from build123d import *

# Parameters (mm, degrees)
SKETCH2_W                                      = 51.0032
SKETCH2_H                                      = 35.1028
BOSS_EXTRUDE1_DEPTH                            = 3.175
BOSS_EXTRUDE3_DEPTH                            = 12.7
M2X0_4_TAPPED_HOLE2_D                          = 1.6
CBORE_FOR_4_SOCKET_HEAD_CAP_SCREW4_D           = 3.2639
CBORE_FOR_4_SOCKET_HEAD_CAP_SCREW4_CBORE_D     = 5.55752
CBORE_FOR_4_SOCKET_HEAD_CAP_SCREW4_CBORE_DEPTH = 12.4968
FILLET1_R                                      = 3.175


with BuildPart() as part:
    # Sketch2 → Boss-Extrude1 (new body)
    with BuildSketch(Plane(origin=(0, 0, 0), x_dir=(1, 0, 0), z_dir=(0, 1, 0))):
        with Locations((-1.5621, -3.9116)):
            Rectangle(SKETCH2_W, SKETCH2_H)
    extrude(amount=BOSS_EXTRUDE1_DEPTH)

    # Sketch14 → Boss-Extrude3 (add)
    with BuildSketch(Plane.XZ):
        Polygon((-27.0637, -13.6398), (-27.0637, 21.463), (23.9395, 21.463), (23.9395, 13.6398), (-19.2405, 13.6398), (-19.2405, -13.6398), align=None)
    extrude(amount=BOSS_EXTRUDE3_DEPTH)

    # M2x0.4 Tapped Hole2 (through all)
    with Locations(Plane(origin=(0, 3.175, 0), x_dir=(1, 0, 0), z_dir=(0, 1, 0))):
        with Locations((-16.3703, 9.0932), (-16.3703, 5.334), (-16.3703, -5.842), (-16.3703, -9.271), (16.5227, -9.271), (16.5227, -5.842), (16.5227, 5.334), (16.5227, 9.0932)):
            Hole(M2X0_4_TAPPED_HOLE2_D / 2)

    # CBORE for #4 Socket Head Cap Screw4 (through all)
    with Locations(Plane(origin=(0, 3.175, 0), x_dir=(1, 0, 0), z_dir=(0, 1, 0))):
        with Locations((-23.1521, 6.8326), (-7.9121, -17.5514), (20.0279, -17.5514)):
            CounterBoreHole(CBORE_FOR_4_SOCKET_HEAD_CAP_SCREW4_D / 2, CBORE_FOR_4_SOCKET_HEAD_CAP_SCREW4_CBORE_D / 2, CBORE_FOR_4_SOCKET_HEAD_CAP_SCREW4_CBORE_DEPTH)

    # Fillet1
    fillet1_edges = [part.edges().sort_by_distance(p)[0] for p in [
        (23.9395, -4.7625, 21.463),
        (23.9395, 1.5875, -13.6398),
        (-27.0637, -4.7625, -13.6398),
        (-27.0637, -4.7625, 21.463),
    ]]
    fillet(fillet1_edges, radius=FILLET1_R)


solid = part.part
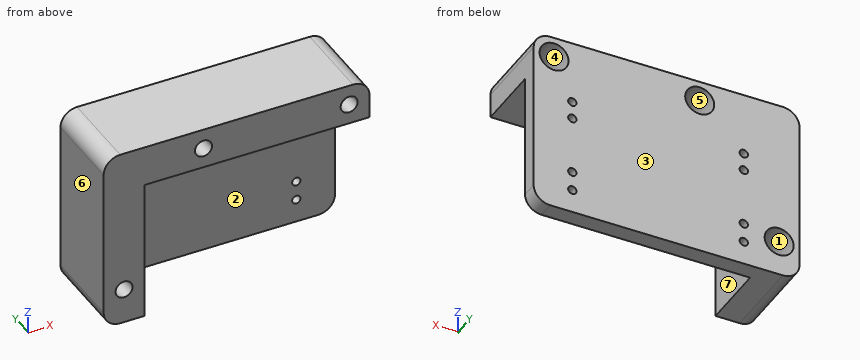
Can you work these out from the model? Positions are in its coordinate system, mm. Face numbers are marked on the shaded views. A direction names the side the tool comes from. Coordinates: 2 decimals unless noted, no trailing zeros. Write each loop counter-clockwise with the first axis right and the second up, starting at its lowest first coordinate (ties: lowest second). Pieces come first, ordered by that corner, then holes. Notation, with made-up numbers: (-37.75, 20.25) -> (12.25, 20.25) arc R30 cw to (12.25, 51.25) -> close; hole circle Ø8 at (-37.5, 82). An arc over 180 degrees is marked (long way). Write each question's results on one line, items separated by ' | '. Start each with the question number.
Item 1: If we section it at C-C, the plane x = 10.5: Write out the boundary of the cut face in (y, z) (3 decimals), and give its area (3 significant figures).
Item 2: If we section it at B-B, the plane x = -7.5: Write out the boundary of the cut face in (y, z) (3 decimals).
Item 3: If we section it at A-A, the plane z = -3.5: Write out the boundary of the cut face in (x, y) (1 decimal).
Item 4: Please list where these lines run through material, in increasing order: probe 1 along Z at (x, y) = (-8, -10); probe 2 along X at (y, z) = (-2, 19); probe 3 along Z at (x, y) = (-18, -1).
Item 5: On a 3-axis mill with a long thin cutter (end or side, diameter ignored), from which of +Z, -Z, +X, -X, +Y, -Y can I reach the whole of each face in a straight line? I mean the marked faces 1, 2 and 3. Say none if no direction works.
Item 6: I'm going to push flat-ended pins straight in: P1, Ø1.3, axis at x = 16.52, z = -9.09, coming from the +Y side; P2, Ø1.5, axis at x = 13.5, z = -1, coming from the -Y side; P3, Ø4, axis at y = -7.5, z = -2, coming from the +X side; P4, Ø4, axis at x = -7.91, z = 17.55, coming from the +Y side. Where does each tip first touch, or does it pass through?
Item 7: If we section it at D-D, the plane y = -6: Count the separate pieces of the cut face and the enclosed holes in it, and give its area (3 significant figures).
Item 8: Thinking about a two-plate mould opening in X: for the marked faces 4, 5, 6 and 7, which applies, released by +X, released by -X, zero draft, split by the parting line, or undercut?
Answer block:
1) outline: (-12.7, 13.64) -> (0, 13.64) -> (0, -13.64) -> (3.175, -13.64) -> (3.175, 21.463) -> (-12.7, 21.463) -> close | area: 211 mm²
2) outline: (-12.7, 13.64) -> (0, 13.64) -> (0, -13.64) -> (3.175, -13.64) -> (3.175, 14.803) -> (-9.322, 14.803) -> (-9.322, 15.972) -> (-12.7, 15.972) -> close; (-12.7, 19.13) -> (-9.322, 19.13) -> (-9.322, 20.299) -> (3.175, 20.299) -> (3.175, 21.463) -> (-12.7, 21.463) -> close
3) outline: (-27.1, -12.7) -> (-19.2, -12.7) -> (-19.2, 0) -> (23.9, 0) -> (23.9, 3.2) -> (-27.1, 3.2) -> close
4) probe 1: 13.64 to 15.92, 19.18 to 21.46 | probe 2: -26.98 to -10.28, -5.54 to 17.66, 22.4 to 23.86 | probe 3: 13.64 to 21.46
5) face 1: +Y | face 2: -Z, +X, -Y | face 3: +Z, -Z, +X, -X, +Y
6) P1: through | P2: y = 0 | P3: x = -19.24 | P4: y = -9.32
7) separate pieces: 1 | enclosed holes: 3 | area: 533 mm²
8) face 4: undercut | face 5: undercut | face 6: released by -X | face 7: released by +X
